Solid Edge part; units mm, degrees
sketch "Sketch1" plane through (0, 0, 0) normal (0, -1, 0) x (1, 0, 0)
  line L0 (25, 0) -> (25, 2)
  arc A0 (23, 4) -> (25, 2) centre (23, 2) cw
  line L1 (23, 4) -> (8, 4)
  arc A1 (4, 8) -> (8, 4) centre (8, 8) ccw
  line L2 (4, 8) -> (4, 38)
  arc A2 (2, 40) -> (4, 38) centre (2, 38) cw
  line L3 (2, 40) -> (0, 40)
  line L4 (0, 40) -> (0, 0)
  line L5 (0, 0) -> (25, 0)
extrude "Protrusion1" add sketch "Sketch1" against normal blind 25.4
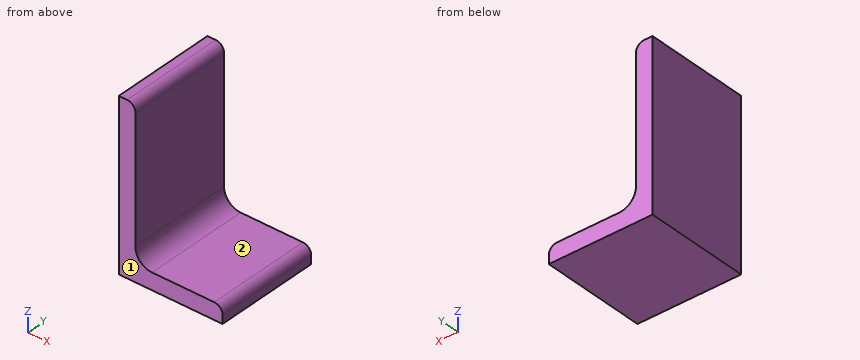
The model under review builds one solid part; all positions refer to its coordinate system, in mm. Face numbers are marked on the shaded views. A direction names the side the tool comes from. Coordinates: 2 decimals unless noted, no trailing zeros. Write each loop counter-clockwise with the first axis right and the second up, starting at its lowest first coordinate (ties: lowest second). Pieces come first, ordered by that corner, then holes.
1) We need section B-B on z = 33.5. State the section outline as (x, y) points.
2) We need section C-C on x = 18.5. State the section outline as (y, z) points, then the cut area to 3 significant figures.
3) To check wall thickness, follow probe 1 along Z at (x, y) = (12.75, 8); probe 2 along X at (y, z) = (8.5, 2.5). State the ranges of each line that lie inside material, in increasing order.
4) Clearance check with flat-ended pins moving along their axes: pin 1 Ø3 at (y, z) = (5, 26.5) entering from +X; pin 2 Ø7.5 at (x, y) = (18.5, 12.5) entering from +Z; pin 3 Ø4 at (x, y) = (7.5, 19.5) entering from +Z. State where each tip first meets the part, or that it passes through.
5) We need section A-A on y = 4. State the section outline as (x, z) points.
6) Machinability: for the marked faces 1 and 2, which of the approach directions +Z, -Z, +X, -X, +Y, -Y give a long, thin tool a straight path to every point of the face, cutting with its end or side? Answer none if there is none.
Answer list:
1. outline: (0, 0) - (4, 0) - (4, 25.4) - (0, 25.4) - close
2. outline: (0, 0) - (25.4, 0) - (25.4, 4) - (0, 4) - close
2. area: 102 mm2
3. probe 1: z = 0 to 4
3. probe 2: x = 0 to 24.94
4. pin 1: stops at x = 4
4. pin 2: stops at z = 4
4. pin 3: stops at z = 4.88
5. outline: (0, 0) - (25, 0) - (25, 2) arc R2 ccw to (23, 4) - (8, 4) arc R4 cw to (4, 8) - (4, 38) arc R2 ccw to (2, 40) - (0, 40) - close
6. face 1: +Z, -Z, +X, -X, -Y
6. face 2: +Z, +X, +Y, -Y
